The model under review builds one solid part; all positions refer to its coordinate system, in mm. A direction names the side the tool comes from. Coordinates: 2 decimals unless noted, no trailing zeros. Write each loop counter-clockwise with the first axis right and the second up, starting at its lowest first coordinate (ties: lowest second). Pieces come first, ordered by that corner, then holes.
```python
from build123d import *


with BuildPart() as f1:
    # F0 (on Front) → F1 (revolve)
    with BuildSketch(Plane.XZ):
        with BuildLine():
            Line((-9.525, 4.7625), (-12.3825, 4.7625))
            ThreePointArc((-12.3825, 4.7625), (-13.729538, 4.204538), (-14.2875, 2.8575))
            Line((-14.2875, 2.8575), (-14.2875, 1.5875))
            Line((-14.2875, 1.5875), (-11.1125, 1.5875))
            Line((-11.1125, 1.5875), (-11.1125, -1.5875))
            Line((-11.1125, -1.5875), (-14.2875, -1.5875))
            Line((-14.2875, -1.5875), (-14.2875, -2.8575))
            ThreePointArc((-14.2875, -2.8575), (-13.729538, -4.204538), (-12.3825, -4.7625))
            Line((-12.3825, -4.7625), (-9.525, -4.7625))
            Line((-9.525, -4.7625), (-9.525, 4.7625))
        make_face()
    revolve(axis=Axis((0, 0, -0.259772), (0, 0, -1)))


solid = f1.part
```
Item 1: To check wall thickness, follow line 1 along Y through (x, z) = (0, -2.5) (1 decimal); line 2 along Z through (x, y) = (-9, 7.5); line 3 along Y through (x, z) = (0, -0.75) (1 decimal). State the ranges of each line that lie inside material, in increasing order.
Solved:
line 1: y = -14.3 to -9.5, 9.5 to 14.3
line 2: z = -4.76 to -1.59, 1.59 to 4.76
line 3: y = -11.1 to -9.5, 9.5 to 11.1
Item 2: Mouldability with a two-part tool opening along Z and no side actions: class faces 1 (the face through (-6.4, -7.3, -4.762)), 2 (the face through (14.274, 0.628, -2.231)), 3 (the face through (6.4, -7.3, 4.762)), 4 (the face through (-10.6, 3.34, -0.02)) as pulls with the +Z half, pulls with the -Z half, needs draft (parallel to the pull), parting line crosses it, or undercut.
Solved:
face 1: pulls with the -Z half
face 2: needs draft
face 3: pulls with the +Z half
face 4: undercut
Item 3: For pin 1 (2 mm diameter, centred on y = 2.5, z = -2.5, fed in from +X); pin 2 (1.5 mm diameter, centred on x = 2.5, z = 3, fed in from +Y); pin 3 (1 mm diameter, centred on x = 1.5, z = -3.5, fed in from -Y), all flat-tipped, find the tip position at first contact; note any pin that passes through.
Solved:
pin 1: stops at x = 14.21
pin 2: stops at y = 14.18
pin 3: stops at y = -14.22
Item 4: Take a section at A-A, the plane x = 0. Write out the cut boundary in (y, z) (1 decimal), plus the area to 3 significant figures.
Solved:
outline: (-14.3, -2.9) arc R1.9 ccw to (-12.4, -4.8) - (-9.5, -4.8) - (-9.5, 4.8) - (-12.4, 4.8) arc R1.9 ccw to (-14.3, 2.9) - (-14.3, 1.6) - (-11.1, 1.6) - (-11.1, -1.6) - (-14.3, -1.6) - close; (9.5, -4.8) - (12.4, -4.8) arc R1.9 ccw to (14.3, -2.9) - (14.3, -1.6) - (11.1, -1.6) - (11.1, 1.6) - (14.3, 1.6) - (14.3, 2.9) arc R1.9 ccw to (12.4, 4.8) - (9.5, 4.8) - close
area: 67.4 mm2
Item 5: Machinability: for faces 5 (the face through (14.274, 0.628, 2.214)), 6 (the face through (9, -7, 1.588)), which of the approach directions +Z, -Z, +X, -X, +Y, -Y give a long, thin tool a straight path to every point of the face, cutting with its end or side? Answer none if there is none.
Solved:
face 5: +Z, -Z
face 6: none
